Autodesk Inventor part; units mm, degrees
ref_plane "YZ Plane" through (0, 0, 0) normal (1, 0, 0) x (0, 1, 0)
ref_plane "XZ Plane" through (0, 0, 0) normal (0, 1, 0) x (-1, 0, 0)
ref_plane "XY Plane" through (0, 0, 0) normal (0, 0, 1) x (1, 0, 0)
sketch "Sketch1" plane through (0, 0, 0) normal (0, 1, 0) x (-1, 0, 0)
  line L0 (0, 0) -> (101.6, 0)
  line L1 (101.6, 0) -> (101.6, 76.2)
  line L2 (101.6, 76.2) -> (0, 76.2)
  line L3 (0, 76.2) -> (0, 0)
  dimension "d0" = 101.6
  dimension "d2" = 76.2
extrude "Plate1" add sketch "Sketch1" along normal blind 3.175
sketch "Sketch2" plane through (-101.6, 3.175, 76.2) normal (-1, 0, 0) x (0, -1, 0)
  line L0 (0, -76.2) -> (0, 0)
  line L1 (0, 0) -> (-47.625, 0)
  line L2 (-47.625, 0) -> (-47.625, -76.2)
  line L3 (-47.625, -76.2) -> (0, -76.2)
edge flange "Flange1" height 50.8 angle 90 thickness 3.175 bend radius 3.175 thickness toward (-1, 0, 0) relief tear relief width 3.175 relief depth 1.5875 edges at (-101.6, 3.175, 38.1) wall of the first edge with corners at (-101.6, 3.175, 0) (-101.6, 3.175, 76.2) (-101.6, 50.8, 76.2) (-101.6, 50.8, 0)
bend "Bend1"
corner "Corner1"
sketch "Sketch3" plane through (0, 3.175, 0) normal (1, 0, 0) x (0, 1, 0)
  line L0 (0, 76.2) -> (0, 0)
  line L1 (0, 0) -> (47.625, 0)
  line L2 (47.625, 0) -> (47.625, 76.2)
  line L3 (47.625, 76.2) -> (0, 76.2)
edge flange "Flange2" height 50.8 angle 90 thickness 3.175 bend radius 3.175 thickness toward (1, 0, 0) relief tear relief width 3.175 relief depth 1.5875 edges at (0, 3.175, 38.1) wall of the first edge with corners at (0, 3.175, 76.2) (0, 3.175, 0) (0, 50.8, 0) (0, 50.8, 76.2)
bend "Bend2"
corner "Corner2"
sketch "Sketch4" plane through (-101.6, 50.8, 76.2) normal (1, 0, 0) x (0, 0, -1)
  line L0 (76.2, 0) -> (0, 0)
  circle A0 centre (44.45, -19.05) radius 14.2875
  point P0 (76.2, -50.8)
  dimension "d24" = 28.575
  dimension "d25" = 19.05
extrude "Cut1" cut sketch "Sketch4" against normal mid plane 5080
sketch "Sketch5" plane through (3.175, 50.8, 76.2) normal (1, 0, 0) x (0, 0, -1)
  circle A0 centre (44.45, -19.05) radius 14.2875
  line L0 (0, -44.45) -> (76.2, -44.45)
  line L1 (76.2, 0) -> (76.2, -44.45)
  line L2 (0, 0) -> (76.2, 0)
  line L3 (0, -44.45) -> (0, 0)
  arc A1 (61.2588, -10.0853) -> (30.6552, -5.9121) centre (44.45, -19.05) ccw
  line L4 (0, -38.1) -> (30.6552, -5.9121)
  line L5 (61.2588, -10.0853) -> (76.2, -38.1)
  point P0 (76.2, -50.8)
  dimension "d28" = 6.35
  dimension "d29" = 6.35
extrude "Cut2" cut sketch "Sketch5" against normal blind 508 contours L3 L2 A1 L4 | L5 A1 L2 L1
sketch "Sketch6" plane through (0, 3.175, 0) normal (0, 1, 0) x (1, 0, 0)
  circle A0 centre (-50.8, -38.1) radius 14.2875
  line L0 (-3.175, -76.2) -> (-3.175, 0)
  line L1 (-3.175, -76.2) -> (-98.425, -76.2)
  point P0 (0, 0)
  dimension "d32" = 28.575
  dimension "d35" = 38.1
  dimension "d36" = 47.625
extrude "Cut3" cut sketch "Sketch6" against normal blind 3.175
equation "\"d33\" = Thickness"
equation "\"d4\" = BendReliefWidth"
equation "\"d5\" = BendReliefDepth"
equation "\"d6\" = MinimumRemnant"
equation "\"d7\" = BendRadius"
equation "\"d10\" = BendRadius"
equation "\"d11\" = CornerReliefSize"
equation "\"d12\" = GapSize"
equation "\"d13\" = JacobiRadiusSize"
equation "\"d14\" = BendReliefWidth"
equation "\"d15\" = BendReliefDepth"
equation "\"d16\" = MinimumRemnant"
equation "\"d17\" = BendRadius"
equation "\"d20\" = BendRadius"
equation "\"d21\" = CornerReliefSize"
equation "\"d22\" = GapSize"
equation "\"d23\" = JacobiRadiusSize"
equation "\"BendRadius\" = Thickness"
equation "\"BendReliefWidth\" = Thickness"
equation "\"BendReliefDepth\" = 0.5 * Thickness"
equation "\"CornerReliefSize\" = 4 * Thickness"
equation "\"MinimumRemnant\" = 2 * Thickness"
equation "\"TransitionRadius\" = BendRadius"
equation "\"JacobiRadiusSize\" = BendRadius"
equation "\"GapSize\" = Thickness"
equation "\"d3\" = BendRadius"
properties part number "Bearing Mount 4 v1" material "Aluminum 6061"
Geometry check sheet. Reference: the model listing, model coordinates, mm. A direction names the side the tool comes from. Give positions to 0.01 mm unless a question says otherwise; leave off trailing zeros. Order: outer loops, then holes, each group sorted by start corner. A loop starts at its lowest first (then second) coordinate and runs counter-clockwise, first axis right, second up. Notation, with made-up numbers: M -37,60 L -21,60 A26 cw -21,88 Z; hole C 22.5,72 d1. An arc over 180 degrees is marked long. Use a Markdown table: item, result.
Item 1: Material ranges on line 1 along X through (y, z) = (7, 9.5) (3 decimals); line 2 along Z through (x, y) = (-50.8, 1.05); line 3 along Y through (x, z) = (-103.6, 31.75), recorded low to high.
Answers follow:
| item | result |
|---|---|
| line 1 | x = -104.775 to -101.6, 0 to 3.175 |
| line 2 | z = 0 to 23.81, 52.39 to 76.2 |
| line 3 | y = 2.67 to 17.46, 46.04 to 50.8 |
Item 2: Tool access check on faces 1 (the cylindrical face through (-103.17, 50.59, 28.93)), 2 (the cylindrical face through (-100.695, 4.13, 38.633)). Record the directions out of +Z, -Z, +X, -X, +Y, -Y that give a thin tool (end or side, any length) a straight path to the whole face; none if there is none.
Answers follow:
| item | result |
|---|---|
| face 1 | +X, -X, +Y |
| face 2 | +Z, -Z, +Y |
Item 3: Section check C-C (y = 31.75). Record the cut outline in (x, z) (1 decimal), and give its area (3 significant figures).
Answers follow:
| item | result |
|---|---|
| outline | M -104.8,10.2 L -101.6,10.2 L -101.6,17.5 L -104.8,17.5 Z; M -104.8,46 L -101.6,46 L -101.6,58.1 L -104.8,58.1 Z; M 0,10.2 L 3.2,10.2 L 3.2,17.5 L 0,17.5 Z; M 0,46 L 3.2,46 L 3.2,58.1 L 0,58.1 Z |
| area | 123 mm2 |
Item 4: Section check A-A (y = 9). Record the cut outline in (x, z) (3 decimals).
Answers follow:
| item | result |
|---|---|
| outline | M -104.775,0 L -101.6,0 L -101.6,76.2 L -104.775,76.2 Z; M 0,0 L 3.175,0 L 3.175,76.2 L 0,76.2 Z |
Item 5: Draft check along X on faces 3 (the flat face through (-51, 2, 0)), 4 (the cylindrical face through (1.364, 1.91, 37.567)), 5 (the cylindrical face through (-0.905, 4.13, 37.567)), 6 (the flat face through (-104.775, 19, 39)). Enter one of: +X half, -X half, draft (parallel to the pull), parting line (faces both ways), or undercut.
Answers follow:
| item | result |
|---|---|
| face 3 | draft |
| face 4 | +X half |
| face 5 | undercut |
| face 6 | -X half |
Item 6: Section check B-B (z = 38.1). State how many separate pieces and enclosed holes the cut face has, and give its area (3 significant figures).
Answers follow:
| item | result |
|---|---|
| separate pieces | 4 |
| enclosed holes | 0 |
| area | 372 mm2 |
Item 7: Depth check by flat-ended pin: P1, Ø1, axis at x = -88, z = 28, coming from the +Y side (3 decimals). Enter the tip coordinate at first touch or a pass-through.
Answers follow:
| item | result |
|---|---|
| P1 | stops at y = 3.175 |
Item 8: Section check D-D (z = 59). Record the cut outline in (x, y) (3 decimals).
Answers follow:
| item | result |
|---|---|
| outline | M -104.775,6.35 A6.35 ccw -98.425,0 L -3.175,0 A6.35 ccw 3.175,6.35 L 3.175,30.76 L 0,30.76 L 0,6.35 A3.175 cw -3.175,3.175 L -98.425,3.175 A3.175 cw -101.6,6.35 L -101.6,30.76 L -104.775,30.76 Z |
